Geometry: final body of the model. Coordinates: model frame, mm. A direction names the side the tool comes from. Give positions to 0.01 mm unless a question says otherwise; leave off trailing zeros. Loops run counter-clockwise (first coordinate to the right, second up) from the corner with the lowest first, then second, coordinate; pieces in that order, holes last. Notation, with made-up numbers: (22, 1) -> (72, 1) arc R14 ccw to (72, 10) -> close; hole circle Ø11 at (20.25, -30.5). An arc over 180 degrees is marked (long way). Answer in a Markdown table with one row per item. Add a question column.
1) Draft query along Y for faces 5 (the flat face through (0, -35.814, 2)), 6 (the flat face through (0, 0, 8.57)), 7 (the flat face through (9.48, -10.34, -7.36)). Return one class per face: +Y half, -Y half, draft (parallel to the pull), parting line (faces both ways), or undercut.
2) Section query C-C (z = 12.5). Return the cut outline in (x, y) (3 decimals), plus the area to 3 significant figures.
3) Access query for faces 1 (the flat face through (0, -23, 3.175)), 2 (the flat face through (0, 0, 15.9)), 3 (the flat face through (0, 2.86, -2)), 4 (the flat face through (0.178, -30.928, -6.327)). Directions: +Z, -Z, +X, -X, +Y, -Y. A direction counts if a zero-diameter tool reaches every point of the face in a straight line with its end or side. Return the directions, or none.
4) First-contact query: P1, Ø8, axis at x = 3.5, z = 16.5, coming from the -Y side (3 decimals); P2, Ø5, axis at x = -1, y = -1.5, coming from the -Z side. Flat tips, straight axial feed; report the tip coordinate or a pass-through.
5) Line query: line 1 (Y direction, x = 0, z = 22.5); line 2 (Y direction, x = 0, z = 21) (3 decimals); line 3 (X direction, y = 0, z = 20). Output: solid intervals per line, ascending. Write a range as from..to.
6) Section query D-D (y = 0). Return the cut outline in (x, z) (3 decimals), plus the area to 3 significant figures.
7) Section query A-A (y = -16). Return the cut outline in (x, z) (3 decimals).
8) Section query B-B (z = 21). Return the cut outline in (x, y) (3 decimals).
```python
from build123d import *

# Parameters (mm, degrees)
BOSS_EXTRUDE1_DEPTH = 25.4
CUT_EXTRUDE1_DEPTH  = 9.5
SKETCH5_W           = 25.4
SKETCH5_H           = 42.164
BOSS_EXTRUDE2_DEPTH = 11.43
CUT_EXTRUDE2_REACH  = 53.538
CUT_EXTRUDE3_REACH  = 53.255
CUT_EXTRUDE4_DEPTH  = 20
SKETCH10_W          = 19.05
SKETCH10_H          = 19.05
CUT_EXTRUDE5_DEPTH  = 26.289
CUT_EXTRUDE6_REACH  = 55.322
SKETCH11_W          = 1.5875
SKETCH11_H          = 12.7


with BuildPart() as part:
    # Sketch2 → Boss-Extrude1 (new body)
    with BuildSketch(Plane.XY):
        Polygon((12.7, -6.35), (14.2875, -6.35), (14.2875, 6.35), (-14.2875, 6.35), (-14.2875, -6.35), (-12.7, -6.35), (-12.7, -35.814), (12.7, -35.814), align=None)
    extrude(amount=BOSS_EXTRUDE1_DEPTH)

    # Sketch3 → Cut-Extrude1 (cut)
    with BuildSketch(Plane.XY.offset(25.4)):
        with BuildLine():
            Line((-2.3, 2.003122562), (2.3, 2.003122562))
            ThreePointArc((2.3, 2.003122562), (0, -3.05), (-2.3, 2.003122562))
        make_face()
    extrude(amount=-CUT_EXTRUDE1_DEPTH, mode=Mode.SUBTRACT)

    # Sketch5 → Boss-Extrude2 (add)
    with BuildSketch(Plane(origin=(0, 0, 0), x_dir=(-1, 0, 0), z_dir=(0, 0, -1))):
        with Locations((0, -14.732)):
            Rectangle(SKETCH5_W, SKETCH5_H)
    extrude(amount=BOSS_EXTRUDE2_DEPTH)

    # Sketch6 → Cut-Extrude2 (cut, up to next)
    with BuildSketch(Plane(origin=(12.7, 0, 0), x_dir=(0, 0, -1), z_dir=(1, 0, 0)), mode=Mode.PRIVATE) as cut_extrude2_sk1:
        Polygon((3.175, -35.814), (11.43, -23.01875), (11.43, -35.814), align=None)
    cut_extrude2_tool1 = extrude(cut_extrude2_sk1.sketch, amount=-CUT_EXTRUDE2_REACH, mode=Mode.PRIVATE) & part.part
    add(cut_extrude2_tool1.solids().sort_by_distance((12.7, -31.548917, -8.678333))[0], mode=Mode.SUBTRACT)

    # Sketch7 → Cut-Extrude3 (cut, up to next)
    with BuildSketch(Plane.XZ.offset(35.814), mode=Mode.PRIVATE) as cut_extrude3_sk1:
        Polygon((-12.7, -11.43), (-12.7, -3.175), (-6.35, -11.43), align=None)
    cut_extrude3_tool1 = extrude(cut_extrude3_sk1.sketch, amount=-CUT_EXTRUDE3_REACH, mode=Mode.PRIVATE) & part.part
    # Sketch7 → Cut-Extrude3 (cut, up to next)
    with BuildSketch(Plane.XZ.offset(35.814), mode=Mode.PRIVATE) as cut_extrude3_sk2:
        Polygon((6.35, -11.43), (12.7, -3.175), (12.7, -11.43), align=None)
    cut_extrude3_tool2 = extrude(cut_extrude3_sk2.sketch, amount=-CUT_EXTRUDE3_REACH, mode=Mode.PRIVATE) & part.part
    add(cut_extrude3_tool1.solids().sort_by_distance((-10.583333, -35.814, -8.678333))[0], mode=Mode.SUBTRACT)
    add(cut_extrude3_tool2.solids().sort_by_distance((10.583333, -35.814, -8.678333))[0], mode=Mode.SUBTRACT)

    # Sketch8 → Cut-Extrude4 (cut)
    with BuildSketch(Plane(origin=(0, 0, -11.43), x_dir=(-1, 0, 0), z_dir=(0, 0, -1))):
        with BuildLine():
            Line((-1.651, 2.859615883), (1.651, 2.859615883))
            ThreePointArc((1.651, 2.859615883), (0, -3.302), (-1.651, 2.859615883))
        make_face()
    extrude(amount=-CUT_EXTRUDE4_DEPTH, mode=Mode.SUBTRACT)

    # Sketch10 → Cut-Extrude5 (cut)
    with BuildSketch(Plane.XZ.offset(35.814)):
        with Locations((0, 12.7)):
            Rectangle(SKETCH10_W, SKETCH10_H)
    extrude(amount=-CUT_EXTRUDE5_DEPTH, mode=Mode.SUBTRACT)

    # Sketch11 → Cut-Extrude6 (cut, up to next)
    with BuildSketch(Plane.XY.offset(25.4), mode=Mode.PRIVATE) as cut_extrude6_sk1:
        with Locations((-13.49375, 0)):
            Rectangle(SKETCH11_W, SKETCH11_H)
    cut_extrude6_tool1 = extrude(cut_extrude6_sk1.sketch, amount=-CUT_EXTRUDE6_REACH, mode=Mode.PRIVATE) & part.part
    # Sketch11 → Cut-Extrude6 (cut, up to next)
    with BuildSketch(Plane.XY.offset(25.4), mode=Mode.PRIVATE) as cut_extrude6_sk2:
        with Locations((13.49375, 0)):
            Rectangle(SKETCH11_W, SKETCH11_H)
    cut_extrude6_tool2 = extrude(cut_extrude6_sk2.sketch, amount=-CUT_EXTRUDE6_REACH, mode=Mode.PRIVATE) & part.part
    add(cut_extrude6_tool1.solids().sort_by_distance((-13.49375, 0, 25.4))[0], mode=Mode.SUBTRACT)
    add(cut_extrude6_tool2.solids().sort_by_distance((13.49375, 0, 25.4))[0], mode=Mode.SUBTRACT)


solid = part.part
```
Evaluation:
| question | item | result |
|---|---|---|
| 1 | face 5 | -Y half |
| 1 | face 6 | undercut |
| 1 | face 7 | draft |
| 2 | outline | (-12.7, -35.814) -> (-9.525, -35.814) -> (-9.525, -9.525) -> (9.525, -9.525) -> (9.525, -35.814) -> (12.7, -35.814) -> (12.7, 6.35) -> (-12.7, 6.35) -> close |
| 2 | area | 570 mm² |
| 3 | face 1 | -Y |
| 3 | face 2 | +Z |
| 3 | face 3 | -Z |
| 3 | face 4 | -Z, +X, -X, -Y |
| 4 | P1 | y = -9.525 |
| 4 | P2 | z = -11.43 |
| 5 | line 1 | -35.81..-3.05, 2..6.35 |
| 5 | line 2 | -9.525..-3.05, 2.003..6.35 |
| 5 | line 3 | -12.7..-3.05, 3.05..12.7 |
| 6 | outline | (-12.7, -3.175) -> (-6.35, -11.43) -> (-3.302, -11.43) -> (-3.302, 8.57) -> (3.302, 8.57) -> (3.302, -11.43) -> (6.35, -11.43) -> (12.7, -3.175) -> (12.7, 25.4) -> (3.05, 25.4) -> (3.05, 15.9) -> (-3.05, 15.9) -> (-3.05, 25.4) -> (-12.7, 25.4) -> close |
| 6 | area | 693 mm² |
| 7 | outline | (-12.7, -3.175) -> (-6.35, -11.43) -> (6.35, -11.43) -> (12.7, -3.175) -> (12.7, 25.4) -> (-12.7, 25.4) -> close; hole (-9.525, 3.175) -> (9.525, 3.175) -> (9.525, 22.225) -> (-9.525, 22.225) -> close |
| 8 | outline | (-12.7, -35.814) -> (-9.525, -35.814) -> (-9.525, -9.525) -> (9.525, -9.525) -> (9.525, -35.814) -> (12.7, -35.814) -> (12.7, 6.35) -> (-12.7, 6.35) -> close; hole (-2.3, 2.003) arc R3.05 ccw (long way) to (2.3, 2.003) -> close |
